from build123d import *

# Parameters (mm, degrees)
F0_W           = 50
F0_H           = 20
F1_DEPTH       = 8
F3_D           = 5.3
F3_CBORE_D     = 10.5
F3_CBORE_DEPTH = 3
F4_W           = 50
F4_H           = 20
F4_W_2         = 47
F4_H_2         = 17
F5_DEPTH       = 1.5


with BuildPart() as f1:
    # F0 (on Top) → F1 (new body)
    with BuildSketch(Plane.XY):
        with Locations((25, 10)):
            Rectangle(F0_W, F0_H)
    extrude(amount=F1_DEPTH)

    # F3 (through all)
    with Locations(Plane.XY.offset(8)):
        with Locations((15, 10), (35, 10)):
            CounterBoreHole(F3_D / 2, F3_CBORE_D / 2, F3_CBORE_DEPTH)

    # F4 (on face) → F5 (join)
    with BuildSketch(Plane.XY.offset(8)):
        with Locations((25, 10)):
            Rectangle(F4_W, F4_H)
        with Locations((25, 10)):
            Rectangle(F4_W_2, F4_H_2, mode=Mode.SUBTRACT)
    extrude(amount=F5_DEPTH)


solid = f1.part
Geometry: final body of the model. Coordinates: model frame, mm. A direction names the side the tool comes from. Give positions to 0.01 mm unless a question says otherwise; leave off trailing zeros. Write each loop counter-clockwise with the first axis right and the second up, starting at its lowest first coordinate (ties: lowest second). Pieces come first, ordered by that corner, then holes.
(1) Cut plane D-D, the plane z = 6. Return loops of the section in (x, y).
(2) First-contact query: P1, Ø4, axis at x = 34, y = 6, coming from the +Z side; P2, Ø1, axis at x = 43, y = 3.5, coming from the -Z side; P3, Ø9.5, axis at x = 35, y = 10, coming from the +Z side; P4, Ø3, axis at x = 15, y = 10, coming from the +Z side. Flat tips, straight axial feed; report the tip coordinate or a pass-through.
(3) Ray query, line 1 (X direction, y = 8, z = 8.25); line 2 (Y direction, x = 15, z = 2.85); line 3 (X direction, y = 11, z = 1.25). Return the intervals inside material, ascending.
(4) Cut plane B-B, the plane y = 10. Return loops of the section in (x, z), then the cut area to 4 significant figures.
(5) Access query for faces 1 (the flat face through (50, 10, 5)), 2 (the flat face through (17, 8, 5)). Directions: +Z, -Z, +X, -X, +Y, -Y. A direction counts if a zero-diameter tool reaches every point of the face in a straight line with its end or side. Return the directions, or none.
(6) Cut plane C-C, the plane z = 8.5. Return loops of the section in (x, y).
(7) Cut plane A-A, the plane x = 35. Return loops of the section in (y, z).
(8) Mould query, pull axis X, two halves, no side actions, for faces 3 (the flat face through (25, 20, 5)), 4 (the cylindrical face through (31.13, 13.55, 6.52)), 5 (the flat face through (0, 10, 5)). Classes: released by +X, released by -X, zero draft, split by the parting line, or undercut.
Values follow:
1. outline: (0, 0) - (50, 0) - (50, 20) - (0, 20) - close; hole circle Ø10.5 at (15, 10); hole circle Ø10.5 at (35, 10)
2. P1: stops at z = 8
2. P2: stops at z = 0
2. P3: stops at z = 5
2. P4: passes through
3. line 1: x = 0 to 1.5, 48.5 to 50
3. line 2: y = 0 to 7.35, 12.65 to 20
3. line 3: x = 0 to 12.55, 17.45 to 32.55, 37.45 to 50
4. outline: (0, 0) - (12.35, 0) - (12.35, 5) - (9.75, 5) - (9.75, 8) - (1.5, 8) - (1.5, 9.5) - (0, 9.5) - close; (17.65, 0) - (32.35, 0) - (32.35, 5) - (29.75, 5) - (29.75, 8) - (20.25, 8) - (20.25, 5) - (17.65, 5) - close; (37.65, 0) - (50, 0) - (50, 9.5) - (48.5, 9.5) - (48.5, 8) - (40.25, 8) - (40.25, 5) - (37.65, 5) - close
4. area: 288.5 mm2
5. face 1: +Z, -Z, +X, +Y, -Y
5. face 2: +Z
6. outline: (0, 0) - (50, 0) - (50, 20) - (0, 20) - close; hole (1.5, 1.5) - (48.5, 1.5) - (48.5, 18.5) - (1.5, 18.5) - close
7. outline: (0, 0) - (7.35, 0) - (7.35, 5) - (4.75, 5) - (4.75, 8) - (1.5, 8) - (1.5, 9.5) - (0, 9.5) - close; (12.65, 0) - (20, 0) - (20, 9.5) - (18.5, 9.5) - (18.5, 8) - (15.25, 8) - (15.25, 5) - (12.65, 5) - close
8. face 3: zero draft
8. face 4: undercut
8. face 5: released by -X
